Work out the finished part from the listing and answer in its coordinate system (mm). Face numbers are marked on the shaded views. A direction names the side the tool comes from. Round coordinates to 2 decimals unless told otherwise and drop trailing zeros. Write each loop counter-clockwise with the first axis right and the second up, starting at its lowest first coordinate (ties: lowest second). Pieces come first, ordered by that corner, then holes. Notation, with made-up numbers: (55, 50) - (112, 50) arc R27 ccw to (112, 80) - close; hole circle Ø9 at (60, 31). An arc over 180 degrees is marked (long way). Answer as a JSON object with one key per item and string values.
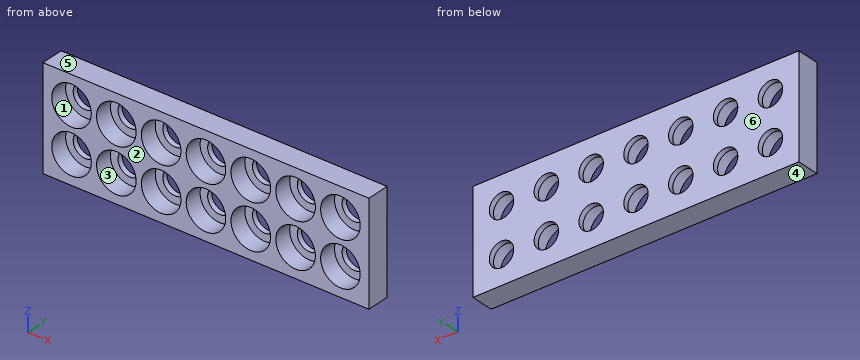
```python
from build123d import *

# Parameters (mm, degrees)
SKETCH3_W           = 186.55
SKETCH3_H           = 58.3
SKETCH3_R           = 11.325
BOSS_EXTRUDE1_DEPTH = 10
BOSS_EXTRUDE3_START = 10
SKETCH3_5_W         = 186.55
SKETCH3_5_H         = 58.3
SKETCH3_5_R         = 11.325
SKETCH3_5_R_2       = 7
BOSS_EXTRUDE3_DEPTH = 3


with BuildPart() as part:
    # Sketch3 → Boss-Extrude1 (new body)
    with BuildSketch(Plane(origin=(0, 0, 0), x_dir=(1, 0, 0), z_dir=(0, 1, 0))):
        with Locations((76.95, 12.825)):
            Rectangle(SKETCH3_W, SKETCH3_H)
        with Locations(Location((0, 25.65, 0), (0, 0, 270))):
            Circle(SKETCH3_R, mode=Mode.SUBTRACT)
        with Locations(Location((153.9, 25.65, 0), (0, 0, 270))):
            Circle(SKETCH3_R, mode=Mode.SUBTRACT)
        with Locations(Location((128.25, 25.65, 0), (0, 0, 270))):
            Circle(SKETCH3_R, mode=Mode.SUBTRACT)
        with Locations(Location((102.6, 25.65, 0), (0, 0, 270))):
            Circle(SKETCH3_R, mode=Mode.SUBTRACT)
        with Locations(Location((76.95, 25.65, 0), (0, 0, 270))):
            Circle(SKETCH3_R, mode=Mode.SUBTRACT)
        with Locations(Location((51.3, 25.65, 0), (0, 0, 270))):
            Circle(SKETCH3_R, mode=Mode.SUBTRACT)
        with Locations(Location((25.65, 25.65, 0), (0, 0, 270))):
            Circle(SKETCH3_R, mode=Mode.SUBTRACT)
        with Locations(Location((153.9, 0, 0), (0, 0, 270))):
            Circle(SKETCH3_R, mode=Mode.SUBTRACT)
        with Locations(Location((128.25, 0, 0), (0, 0, 270))):
            Circle(SKETCH3_R, mode=Mode.SUBTRACT)
        with Locations(Location((102.6, 0, 0), (0, 0, 270))):
            Circle(SKETCH3_R, mode=Mode.SUBTRACT)
        with Locations(Location((76.95, 0, 0), (0, 0, 270))):
            Circle(SKETCH3_R, mode=Mode.SUBTRACT)
        with Locations(Location((51.3, 0, 0), (0, 0, 270))):
            Circle(SKETCH3_R, mode=Mode.SUBTRACT)
        with Locations(Location((25.65, 0, 0), (0, 0, 270))):
            Circle(SKETCH3_R, mode=Mode.SUBTRACT)
        with Locations(Location((0, 0, 0), (0, 0, 270))):
            Circle(SKETCH3_R, mode=Mode.SUBTRACT)
    extrude(amount=BOSS_EXTRUDE1_DEPTH)

    # Sketch3_5 → Boss-Extrude3 (add)
    # profile 1 of 15: a face of its own
    with BuildSketch(Plane(origin=(0, 0, 0), x_dir=(1, 0, 0), z_dir=(0, 1, 0)).offset(BOSS_EXTRUDE3_START)):
        with Locations((76.95, 12.825)):
            Rectangle(SKETCH3_5_W, SKETCH3_5_H)
        with Locations(Location((0, 25.65, 0), (0, 0, 270))):
            Circle(SKETCH3_5_R, mode=Mode.SUBTRACT)
        with Locations(Location((153.9, 25.65, 0), (0, 0, 270))):
            Circle(SKETCH3_5_R, mode=Mode.SUBTRACT)
        with Locations(Location((128.25, 25.65, 0), (0, 0, 270))):
            Circle(SKETCH3_5_R, mode=Mode.SUBTRACT)
        with Locations(Location((102.6, 25.65, 0), (0, 0, 270))):
            Circle(SKETCH3_5_R, mode=Mode.SUBTRACT)
        with Locations(Location((76.95, 25.65, 0), (0, 0, 270))):
            Circle(SKETCH3_5_R, mode=Mode.SUBTRACT)
        with Locations(Location((51.3, 25.65, 0), (0, 0, 270))):
            Circle(SKETCH3_5_R, mode=Mode.SUBTRACT)
        with Locations(Location((25.65, 25.65, 0), (0, 0, 270))):
            Circle(SKETCH3_5_R, mode=Mode.SUBTRACT)
        with Locations(Location((153.9, 0, 0), (0, 0, 270))):
            Circle(SKETCH3_5_R, mode=Mode.SUBTRACT)
        with Locations(Location((128.25, 0, 0), (0, 0, 270))):
            Circle(SKETCH3_5_R, mode=Mode.SUBTRACT)
        with Locations(Location((102.6, 0, 0), (0, 0, 270))):
            Circle(SKETCH3_5_R, mode=Mode.SUBTRACT)
        with Locations(Location((76.95, 0, 0), (0, 0, 270))):
            Circle(SKETCH3_5_R, mode=Mode.SUBTRACT)
        with Locations(Location((51.3, 0, 0), (0, 0, 270))):
            Circle(SKETCH3_5_R, mode=Mode.SUBTRACT)
        with Locations(Location((25.65, 0, 0), (0, 0, 270))):
            Circle(SKETCH3_5_R, mode=Mode.SUBTRACT)
        with Locations(Location((0, 0, 0), (0, 0, 270))):
            Circle(SKETCH3_5_R, mode=Mode.SUBTRACT)
    # profile 2 of 15: a face of its own
    with BuildSketch(Plane(origin=(0, 0, 0), x_dir=(1, 0, 0), z_dir=(0, 1, 0)).offset(BOSS_EXTRUDE3_START)):
        with Locations(Location((153.9, 0, 0), (0, 0, 270))):
            Circle(SKETCH3_5_R)
        with Locations(Location((153.9, 0, 0), (0, 0, 270))):
            Circle(SKETCH3_5_R_2, mode=Mode.SUBTRACT)
    # profile 3 of 15: a face of its own
    with BuildSketch(Plane(origin=(0, 0, 0), x_dir=(1, 0, 0), z_dir=(0, 1, 0)).offset(BOSS_EXTRUDE3_START)):
        with Locations(Location((153.9, 25.65, 0), (0, 0, 270))):
            Circle(SKETCH3_5_R)
        with Locations(Location((153.9, 25.65, 0), (0, 0, 270))):
            Circle(SKETCH3_5_R_2, mode=Mode.SUBTRACT)
    # profile 4 of 15: a face of its own
    with BuildSketch(Plane(origin=(0, 0, 0), x_dir=(1, 0, 0), z_dir=(0, 1, 0)).offset(BOSS_EXTRUDE3_START)):
        with Locations(Location((128.25, 0, 0), (0, 0, 270))):
            Circle(SKETCH3_5_R)
        with Locations(Location((128.25, 0, 0), (0, 0, 270))):
            Circle(SKETCH3_5_R_2, mode=Mode.SUBTRACT)
    # profile 5 of 15: a face of its own
    with BuildSketch(Plane(origin=(0, 0, 0), x_dir=(1, 0, 0), z_dir=(0, 1, 0)).offset(BOSS_EXTRUDE3_START)):
        with Locations(Location((128.25, 25.65, 0), (0, 0, 270))):
            Circle(SKETCH3_5_R)
        with Locations(Location((128.25, 25.65, 0), (0, 0, 270))):
            Circle(SKETCH3_5_R_2, mode=Mode.SUBTRACT)
    # profile 6 of 15: a face of its own
    with BuildSketch(Plane(origin=(0, 0, 0), x_dir=(1, 0, 0), z_dir=(0, 1, 0)).offset(BOSS_EXTRUDE3_START)):
        with Locations(Location((102.6, 0, 0), (0, 0, 270))):
            Circle(SKETCH3_5_R)
        with Locations(Location((102.6, 0, 0), (0, 0, 270))):
            Circle(SKETCH3_5_R_2, mode=Mode.SUBTRACT)
    # profile 7 of 15: a face of its own
    with BuildSketch(Plane(origin=(0, 0, 0), x_dir=(1, 0, 0), z_dir=(0, 1, 0)).offset(BOSS_EXTRUDE3_START)):
        with Locations(Location((102.6, 25.65, 0), (0, 0, 270))):
            Circle(SKETCH3_5_R)
        with Locations(Location((102.6, 25.65, 0), (0, 0, 270))):
            Circle(SKETCH3_5_R_2, mode=Mode.SUBTRACT)
    # profile 8 of 15: a face of its own
    with BuildSketch(Plane(origin=(0, 0, 0), x_dir=(1, 0, 0), z_dir=(0, 1, 0)).offset(BOSS_EXTRUDE3_START)):
        with Locations(Location((76.95, 0, 0), (0, 0, 270))):
            Circle(SKETCH3_5_R)
        with Locations(Location((76.95, 0, 0), (0, 0, 270))):
            Circle(SKETCH3_5_R_2, mode=Mode.SUBTRACT)
    # profile 9 of 15: a face of its own
    with BuildSketch(Plane(origin=(0, 0, 0), x_dir=(1, 0, 0), z_dir=(0, 1, 0)).offset(BOSS_EXTRUDE3_START)):
        with Locations(Location((76.95, 25.65, 0), (0, 0, 270))):
            Circle(SKETCH3_5_R)
        with Locations(Location((76.95, 25.65, 0), (0, 0, 270))):
            Circle(SKETCH3_5_R_2, mode=Mode.SUBTRACT)
    # profile 10 of 15: a face of its own
    with BuildSketch(Plane(origin=(0, 0, 0), x_dir=(1, 0, 0), z_dir=(0, 1, 0)).offset(BOSS_EXTRUDE3_START)):
        with Locations(Location((51.3, 0, 0), (0, 0, 270))):
            Circle(SKETCH3_5_R)
        with Locations(Location((51.3, 0, 0), (0, 0, 270))):
            Circle(SKETCH3_5_R_2, mode=Mode.SUBTRACT)
    # profile 11 of 15: a face of its own
    with BuildSketch(Plane(origin=(0, 0, 0), x_dir=(1, 0, 0), z_dir=(0, 1, 0)).offset(BOSS_EXTRUDE3_START)):
        with Locations(Location((51.3, 25.65, 0), (0, 0, 270))):
            Circle(SKETCH3_5_R)
        with Locations(Location((51.3, 25.65, 0), (0, 0, 270))):
            Circle(SKETCH3_5_R_2, mode=Mode.SUBTRACT)
    # profile 12 of 15: a face of its own
    with BuildSketch(Plane(origin=(0, 0, 0), x_dir=(1, 0, 0), z_dir=(0, 1, 0)).offset(BOSS_EXTRUDE3_START)):
        with Locations(Location((25.65, 0, 0), (0, 0, 270))):
            Circle(SKETCH3_5_R)
        with Locations(Location((25.65, 0, 0), (0, 0, 270))):
            Circle(SKETCH3_5_R_2, mode=Mode.SUBTRACT)
    # profile 13 of 15: a face of its own
    with BuildSketch(Plane(origin=(0, 0, 0), x_dir=(1, 0, 0), z_dir=(0, 1, 0)).offset(BOSS_EXTRUDE3_START)):
        with Locations(Location((25.65, 25.65, 0), (0, 0, 270))):
            Circle(SKETCH3_5_R)
        with Locations(Location((25.65, 25.65, 0), (0, 0, 270))):
            Circle(SKETCH3_5_R_2, mode=Mode.SUBTRACT)
    # profile 14 of 15: a face of its own
    with BuildSketch(Plane(origin=(0, 0, 0), x_dir=(1, 0, 0), z_dir=(0, 1, 0)).offset(BOSS_EXTRUDE3_START)):
        with Locations(Location((0, 0, 0), (0, 0, 270))):
            Circle(SKETCH3_5_R)
        with Locations(Location((0, 0, 0), (0, 0, 270))):
            Circle(SKETCH3_5_R_2, mode=Mode.SUBTRACT)
    # profile 15 of 15: a face of its own
    with BuildSketch(Plane(origin=(0, 0, 0), x_dir=(1, 0, 0), z_dir=(0, 1, 0)).offset(BOSS_EXTRUDE3_START)):
        with Locations(Location((0, 25.65, 0), (0, 0, 270))):
            Circle(SKETCH3_5_R)
        with Locations(Location((0, 25.65, 0), (0, 0, 270))):
            Circle(SKETCH3_5_R_2, mode=Mode.SUBTRACT)
    extrude(amount=BOSS_EXTRUDE3_DEPTH)


solid = part.part
```
Item 1: For the marked faces 1 and 2, determine the directions among +Z, -Z, +X, -X, +Y, -Y from which every point of the face is accessible in a straight line to the end or side of a thin tool.
Results found:
{"face 1": "-Y", "face 2": "+Z, -Z, +X, -X, -Y"}
Item 2: A cutting plane is placed at D-D (x = 108). Write down the section's boundary in (y, z) (3 decimals).
Results found:
{"outline": "(0, -41.975) - (13, -41.975) - (13, -30.104) - (10, -30.104) - (10, -35.605) - (0, -35.605) - close; (0, -15.695) - (10, -15.695) - (10, -21.196) - (13, -21.196) - (13, -4.454) - (10, -4.454) - (10, -9.955) - (0, -9.955) - close; (0, 9.955) - (10, 9.955) - (10, 4.454) - (13, 4.454) - (13, 16.325) - (0, 16.325) - close"}
Item 3: A cutting plane is placed at B-B (y = 7.5). Give the number of separate pieces and of enclosed holes in the cut face, and give its area (3 significant figures).
Results found:
{"separate pieces": "1", "enclosed holes": "14", "area": "5,230 mm²"}
Item 4: Consider line 1 along Z through (x, y) = (125, 4.75) (3 decimals); line 2 along Z through (x, y) = (22, 12.75) (3 decimals); line 3 along Y through (x, z) = (25, -15). Determine where each line is inside the solid, lowest interval first.
Results found:
{"line 1": "-41.975 to -36.499, -14.801 to -10.849, 10.849 to 16.325", "line 2": "-41.975 to -31.623, -19.677 to -5.973, 5.973 to 16.325", "line 3": "10 to 13"}
Item 5: A cutting plane is placed at A-A (x = 51.3). Write down the section's boundary in (y, z) (3 decimals), and give its area (3 significant figures).
Results found:
{"outline": "(0, -41.975) - (13, -41.975) - (13, -32.65) - (10, -32.65) - (10, -36.975) - (0, -36.975) - close; (0, -14.325) - (10, -14.325) - (10, -18.65) - (13, -18.65) - (13, -7) - (10, -7) - (10, -11.325) - (0, -11.325) - close; (0, 11.325) - (10, 11.325) - (10, 7) - (13, 7) - (13, 16.325) - (0, 16.325) - close", "area": "221 mm²"}
Item 6: This flat-tipped pin is pushed along its axis until it touches: P1, Ø1, axis at x = 55.5, z = 6, coming from the -Y side. Where does it stop, or does it pass through?
Results found:
{"P1": "y = 10"}
Item 7: Determine the mould class of the marked faces 3, 4, 5 and 6 for opening direction Z: pulls with the +Z half, pulls with the -Z half, needs draft (parallel to the pull), parting line crosses it, or undercut.
Results found:
{"face 3": "undercut", "face 4": "pulls with the -Z half", "face 5": "pulls with the +Z half", "face 6": "needs draft"}
